Geometry check sheet. Reference: the model listing, model coordinates, mm. Coordinates: 2 decimals unless noted, no trailing zeros. Order: outer loops, then holes, each group sorted by start corner. A loop starts at its lowest first (then second) coordinate and runs counter-clockwise, first axis right, second up. Notation, with made-up numbers: (45.25, -1) - (96.25, -1) arc R27 ccw to (96.25, 27) - close; hole circle Ø10 at (-12.75, 89). An arc over 180 degrees is marked (long way). Return JSON: item names as keys, results as strings. Group by question number.
Item 1: Section check B-B on z = 53. Enter the section's corners in (x, y), then the cut area to 3 significant figures.
Item 2: Scan lines: probe 1 along Y at (x, z) = (732, -20.5); probe 2 along X at (y, z) = (36, 86.5); probe 3 along X at (y, z) = (38.5, 50.5). Record each from-to range of solid material in increasing order.
Item 3: Gauge pin test, flat ends, axial feed: pin 1 (2 mm diameter, centred on x = -663, z = -27, fed in from +Y); pin 2 (4 mm diameter, centred on x = 551.5, y = 13, fed in from -Z); pin 3 (2 mm diameter, centred on x = -457.5, y = 31, fed in from +Z). Record the tip position at first contact, or that the pin passes through.
Item 4: Section check D-D on z = -84. Enter the section's corners in (x, y), then the cut area to 3 significant figures.
Item 5: Section check A-A on x = -524.5. Enter the section's corners in (y, z), then the cut area to 3 significant figures.
Item 6: Section check C-C on y = 16. Enter the section's corners in (x, z), then the cut area to 3 significant figures.
from build123d import *

# Parameters (mm, degrees)
SKETCH1_W           = 2400
SKETCH1_H           = 225
BOSS_EXTRUDE1_DEPTH = 10
BOSS_EXTRUDE2_START = 30
BOSS_EXTRUDE2_DEPTH = 80
BOSS_EXTRUDE3_START = -30
BOSS_EXTRUDE3_DEPTH = 80


with BuildPart() as part:
    # Sketch1 → Boss-Extrude1 (new body)
    with BuildSketch(Plane(origin=(0, 0, 0), x_dir=(1, 0, 0), z_dir=(0, 1, 0))):
        Rectangle(SKETCH1_W, SKETCH1_H)
    extrude(amount=BOSS_EXTRUDE1_DEPTH)

    # Sketch2 → Boss-Extrude2 (add)
    with BuildSketch(Plane.XY.offset(BOSS_EXTRUDE2_START)):
        Polygon((600, 10), (579.09266135, 40), (454.09266135, 40), (425, 10), align=None)
        Polygon((-420.90733865, 40), (-545.90733865, 40), (-575, 10), (-400, 10), align=None)
    extrude(amount=BOSS_EXTRUDE2_DEPTH)

    # Sketch4 → Boss-Extrude3 (add)
    with BuildSketch(Plane.XY.offset(BOSS_EXTRUDE3_START)):
        Polygon((100, 10), (79.09266135, 40), (-45.90733865, 40), (-75, 10), align=None)
    extrude(amount=-BOSS_EXTRUDE3_DEPTH)


solid = part.part
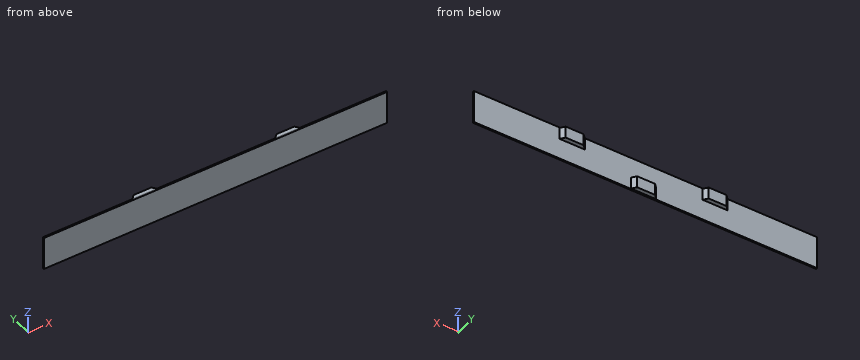
Computed:
{
 "1": {"outline": "(-1200, 0) - (1200, 0) - (1200, 10) - (600, 10) - (579.09, 40) - (454.09, 40) - (425, 10) - (-400, 10) - (-420.91, 40) - (-545.91, 40) - (-575, 10) - (-1200, 10) - close", "area": "33,000 mm²"},
 "2": {"probe 1": "y = 0 to 10", "probe 2": "x = -549.79 to -418.12, 450.21 to 581.88", "probe 3": "x = -547.36 to -419.86, 452.64 to 580.14"},
 "3": {"pin 1": "stops at y = 10", "pin 2": "stops at z = 30", "pin 3": "stops at z = 110"},
 "4": {"outline": "(-1200, 0) - (1200, 0) - (1200, 10) - (100, 10) - (79.09, 40) - (-45.91, 40) - (-75, 10) - (-1200, 10) - close", "area": "28,500 mm²"},
 "5": {"outline": "(0, -112.5) - (10, -112.5) - (10, 30) - (40, 30) - (40, 110) - (10, 110) - (10, 112.5) - (0, 112.5) - close", "area": "4,650 mm²"},
 "6": {"outline": "(-569.18, 30) - (-404.18, 30) - (-404.18, 110) - (-569.18, 110) - close; (-69.18, -110) - (95.82, -110) - (95.82, -30) - (-69.18, -30) - close; (430.82, 30) - (595.82, 30) - (595.82, 110) - (430.82, 110) - close", "area": "39,600 mm²"}
}
